Geometry check sheet. Reference: the model listing, model coordinates, mm. Face numbers are marked on the shaded views. A direction names the side the tool comes from. Give positions to 0.01 mm unless a question says otherwise; leave off trailing zeros. Write each loop counter-clockwise with the first axis right and the second up, starting at its lowest first coordinate (ties: lowest second). Pieces come first, ordered by that corner, then holes. Notation, with made-up numbers: (75.25, 6) - (123.25, 6) arc R27 ccw to (123.25, 33) - close; hole circle Ø1 at (11, -21). An arc over 180 degrees is marked (long way). Use a Markdown table: item, result.
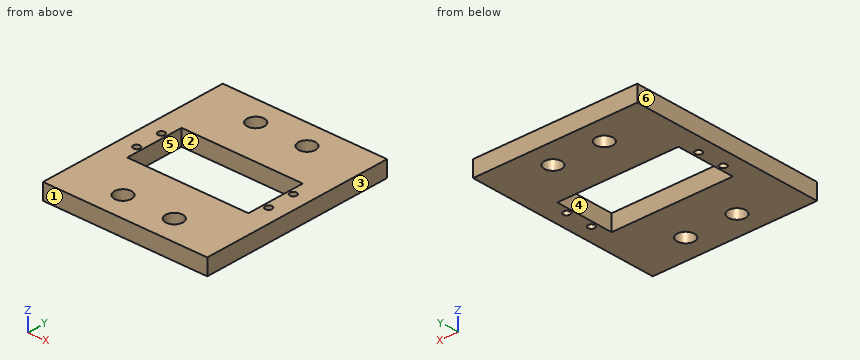
```python
from build123d import *

# Parameters (mm, degrees)
SKETCH1_W           = 61
SKETCH1_H           = 72.8
SKETCH1_R           = 1.27
SKETCH1_R_2         = 3.175
SKETCH1_W_2         = 45
SKETCH1_H_2         = 22
BOSS_EXTRUDE1_DEPTH = 5.9944


with BuildPart() as part:
    # Sketch1 → Boss-Extrude1 (new body)
    with BuildSketch(Plane.XY):
        with Locations((22.5, 11)):
            Rectangle(SKETCH1_W, SKETCH1_H)
        with Locations((-2, 16)):
            Circle(SKETCH1_R, mode=Mode.SUBTRACT)
        with Locations((-2, 6)):
            Circle(SKETCH1_R, mode=Mode.SUBTRACT)
        with Locations((47, 16)):
            Circle(SKETCH1_R, mode=Mode.SUBTRACT)
        with Locations((47, 6)):
            Circle(SKETCH1_R, mode=Mode.SUBTRACT)
        with Locations((12.975, -15.875)):
            Circle(SKETCH1_R_2, mode=Mode.SUBTRACT)
        with Locations((12.975, 37.875)):
            Circle(SKETCH1_R_2, mode=Mode.SUBTRACT)
        with Locations((32.025, 37.875)):
            Circle(SKETCH1_R_2, mode=Mode.SUBTRACT)
        with Locations((32.025, -15.875)):
            Circle(SKETCH1_R_2, mode=Mode.SUBTRACT)
        with Locations((22.5, 11)):
            Rectangle(SKETCH1_W_2, SKETCH1_H_2, mode=Mode.SUBTRACT)
    extrude(amount=BOSS_EXTRUDE1_DEPTH)


solid = part.part
```
1) Section check B-B on y = 6. Record the boundary of the cut face in (x, z).
Working result:
| item | result |
|---|---|
| outline | (-8, 0) - (-3.27, 0) - (-3.27, 5.99) - (-8, 5.99) - close; (-0.73, 0) - (0, 0) - (0, 5.99) - (-0.73, 5.99) - close; (45, 0) - (45.73, 0) - (45.73, 5.99) - (45, 5.99) - close; (48.27, 0) - (53, 0) - (53, 5.99) - (48.27, 5.99) - close |
2) Mould release check, pull along X, two halves, no side actions. Record for the marked faces 3, 4, 5 and 6: pulls with the +X half, pulls with the -X half, needs draft (parallel to the pull), parting line crosses it, or undercut.
Working result:
| item | result |
|---|---|
| face 3 | pulls with the +X half |
| face 4 | undercut |
| face 5 | undercut |
| face 6 | pulls with the -X half |
3) Section check A-A on x = 36. Record the boundary of the cut face in (y, z), then the cut area to 3 significant figures.
Working result:
| item | result |
|---|---|
| outline | (-25.4, 0) - (0, 0) - (0, 5.99) - (-25.4, 5.99) - close; (22, 0) - (47.4, 0) - (47.4, 5.99) - (22, 5.99) - close |
| area | 305 mm² |
4) Set-up check for the marked faces 1 and 2: record each of +Z, -Z, +X, -X, +Y, -Y from which the full face is reachable in a straight line by a thin tool's end or side.
Working result:
| item | result |
|---|---|
| face 1 | +Z, -Z, +X, -X, -Y |
| face 2 | +Z, -Z |
5) Depth check by flat-ended pin: P1, Ø5, axis at x = 32.025, y = -15.875, coming from the +Z side. Enter the tip coordinate at first touch or a pass-through.
Working result:
| item | result |
|---|---|
| P1 | passes through |
6) Material ranges on L1, parallel to Y at x = -2, z = 2.05; L2, parallel to Y at x = 20, z = 1.25; L3, parallel to X at y = 17, z = 3.3, recorded low to high. Write a range as from..to.
Working result:
| item | result |
|---|---|
| L1 | y = -25.4..4.73, 7.27..14.73, 17.27..47.4 |
| L2 | y = -25.4..0, 22..47.4 |
| L3 | x = -8..-2.78, -1.22..0, 45..46.22, 47.78..53 |
7) Section check D-D on z = 2.5. Count the separate pieces of the cut face and the enclosed holes in it, then the cut area to 3 significant figures.
Working result:
| item | result |
|---|---|
| separate pieces | 1 |
| enclosed holes | 9 |
| area | 3,300 mm² |
8) Section check C-C on x = 47. Record the boundary of the cut face in (y, z).
Working result:
| item | result |
|---|---|
| outline | (-25.4, 0) - (4.73, 0) - (4.73, 5.99) - (-25.4, 5.99) - close; (7.27, 0) - (14.73, 0) - (14.73, 5.99) - (7.27, 5.99) - close; (17.27, 0) - (47.4, 0) - (47.4, 5.99) - (17.27, 5.99) - close |
